Design review of the part built by this model. Coordinates are the model's own, in mm. A direction names the side the tool comes from. Coordinates: 2 decimals unless noted, no trailing zeros. Order: outer loops, then holes, each group sorted by start corner. A loop starts at its lowest first (then second) coordinate and runs counter-clockwise, first axis right, second up. Notation, with made-up numbers: M 39.25,8.5 L 75.25,8.5 A16 cw 75.25,27.5 Z; hole C -19,69.25 d1. An arc over 180 degrees is marked long. Use CSV: the item, a comma, the result in double quotes.
```python
from build123d import *

# Parameters (mm, degrees)
F0_W     = 60
F0_H     = 90
F1_DEPTH = 15
F2_W     = 20
F2_H     = 30
F3_DEPTH = 15
F5_DEPTH = 60
F6_W     = 20
F6_H     = 30
F7_DEPTH = 15


with BuildPart() as f1:
    # F0 (on Top) → F1 (new body)
    with BuildSketch(Plane.XY):
        with Locations((-30, 43.088234)):
            Rectangle(F0_W, F0_H)
    extrude(amount=F1_DEPTH)

    # F2 (on face) → F3 (join)
    with BuildSketch(Plane.XY.offset(15)):
        with Locations((-50, 73.088234)):
            Rectangle(F2_W, F2_H)
        with Locations((-10, 73.088234)):
            Rectangle(F2_W, F2_H)
    extrude(amount=F3_DEPTH)

    # F4 (on face) → F5 (cut)
    with BuildSketch(Plane.YZ):
        Polygon((-1.911766, 15), (-1.911766, 0), (28.088234, 15), align=None)
    extrude(amount=-F5_DEPTH, mode=Mode.SUBTRACT)

    # F6 (on face) → F7 (cut)
    with BuildSketch(Plane(origin=(0, 0, 0), x_dir=(1, 0, 0), z_dir=(0, 0, -1))):
        with Locations((-30, -13.088234)):
            Rectangle(F6_W, F6_H)
    extrude(amount=-F7_DEPTH, mode=Mode.SUBTRACT)


solid = f1.part
```
(1) Add section A-A on z = 25.25. State the section outline as (x, y) points, and give its area (3 significant figures).
The answers:
outline,"M -60,58.09 L -40,58.09 L -40,88.09 L -60,88.09 Z; M -20,58.09 L 0,58.09 L 0,88.09 L -20,88.09 Z"
area,"1,200 mm2"
(2) Add section D-D on z = 4.5. State the section outline as (x, y) points.
The answers:
outline,"M -60,7.09 L -40,7.09 L -40,28.09 L -20,28.09 L -20,7.09 L 0,7.09 L 0,88.09 L -60,88.09 Z"
(3) The part is to be moulded in two halves that separate along X. For faces 1 (the face through (-9.86, 12.878, 7.395)), 2 (the face through (-30, 52, 15)), 3 (the face through (-60, 52, 11)), say which applies: pulls with the +X half, pulls with the -X half, needs draft (parallel to the pull), parting line crosses it, or undercut.
The answers:
face 1,"needs draft"
face 2,"undercut"
face 3,"pulls with the -X half"
(4) Clearance check with flat-ended pins moving along their axes: P1, Ø7.5, axis at x = -29.5, z = 6, coming from the -Y side; P2, Ø5, axis at x = -14.5, z = 12, coming from the -Y side; P3, Ø16.5, axis at x = -12, z = 22.5, coming from the -Y side. State where each tip first meets the part, or that it passes through.
The answers:
P1,"stops at y = 28.09"
P2,"stops at y = 17.09"
P3,"stops at y = 26.59"
(5) Wall thickness on probe 1 along X at (y, z) = (79, 26.25); probe 2 along Z at (x, y) = (-20, 38); probe 3 along Y at (x, z) = (-34, 5): over which ranges is each line inside the solid? List them lowest first.
The answers:
probe 1,"x = -60 to -40, -20 to 0"
probe 2,"z = 0 to 15"
probe 3,"y = 28.09 to 88.09"
(6) Add section B-B on y = 9. State the section outline as (x, z) points.
The answers:
outline,"M -60,0 L -40,0 L -40,5.46 L -60,5.46 Z; M -20,0 L 0,0 L 0,5.46 L -20,5.46 Z"
(7) For faces 4 (the face through (-50, 58.088, 22)), 5 (the face through (-30, 28.088, 7)), 6 (the face through (-40, 73, 22)), list the 3-axis set-ups (+Z, -Z, +X, -X, +Y, -Y) from which the entire face can be reached by the end or side of a thin tool; tool diameter is ignored.
The answers:
face 4,"+Z, +X, -X, -Y"
face 5,"+Z, -Z, -Y"
face 6,"+Z, +Y, -Y"
(8) Add section C-C on x = -51. State the section outline as (y, z) points.
The answers:
outline,"M -1.91,0 L 88.09,0 L 88.09,30 L 58.09,30 L 58.09,15 L 28.09,15 Z"
